Geometry: final body of the model. Coordinates: model frame, mm. A direction names the side the tool comes from. Coordinates: 2 decimals unless noted, no trailing zeros. Write each loop counter-clockwise with the first axis right and the second up, starting at its lowest first coordinate (ties: lowest second). Pieces come first, ordered by that corner, then holes. Notation, with made-up numbers: M 68,22.25 L 83,22.25 A22 cw 83,51.25 Z; hole C 89,66 d11. An arc over 180 degrees is marked long. Write item = value, one per line. Start each with the question number.
Item 1: First-contact query: pin 1 Ø10 at (x, z) = (4, -7.5) entering from -Y; pin 2 Ø8 at (x, z) = (-5, -3) entering from -Y; pin 3 Ø2 at (x, z) = (14.5, 0.5) entering from -Y; pin 4 Ø1.6 at (x, z) = (17, 6) entering from -Y. Flat tips, straight axial feed; report the tip coordinate or a pass-through.
Item 2: Section C-C on x = -9. Output: boundary loops of the cut face in (y, z) (3 decimals).
Item 3: Reachability of faces 4 (the flat face through (0, 2, 0)), 5 (the flat face through (0, 5, 12.925)), 6 (the flat face through (15.72, 0.99, -0.18)) from +Z, -Z, +X, -X, +Y, -Y: full face, straight path, thin tool, end or side. Return the list, or none.
Item 4: Section A-A on y = -3. Give the number of separate pieces and of enclosed holes in the cut face, plus the area to 3 significant figures.
Item 5: Pull-direction query (X, two-part tool) for faces 1 (the flat face through (-15.704, 1.014, -0.181)), 2 (the flat face through (-17.9, 4, 0)), 3 (the flat face through (0, 5, -12.925)); classes: +X half, -X half, draft (parallel to the pull), parting line (faces both ways), or undercut.
Item 6: Ray query, L1, parallel to Y at x = 2, z = -4; L2, parallel to X at y = 1.75, z = 7.75; L3, parallel to X at y = 0.75, z = -4.25. Return the intervals inside material, ascending. Write a range as [from, to].
Item 7: Section B-B on z = -5.75. Output: boundary loops of the cut face in (x, y), plus the area to 3 significant figures.
from build123d import *

# Parameters (mm, degrees)
SKETCH_1_W                  = 35.8
SKETCH_1_H                  = 25.85
EXTRUDE_1_DEPTH             = 7.74
CUT_EXTRUDE_1_DEPTH         = 33.38116891
CUT_EXTRUDE_1_DEPTH_BACK    = 33.38116891
SKETCH_1_4_R                = 0.25
EXTRUDE_2_DEPTH             = 4
EXTRUDE_2_DIRECTION_2_REACH = 25.396


with BuildPart() as part:
    # Sketch 1 → Extrude 1 (new body)
    with BuildSketch(Plane(origin=(0, 0, 0), x_dir=(1, 0, 0), z_dir=(0, 1, 0))):
        Rectangle(SKETCH_1_W, SKETCH_1_H)
    extrude(amount=EXTRUDE_1_DEPTH)

    # Sketch 2 → Cut-Extrude 1 (cut, two sides: drawn at the far end of the back side and taken through both)
    with BuildSketch(Plane.XY.offset(12.925).offset(-CUT_EXTRUDE_1_DEPTH_BACK)):
        Polygon((-15.027609673, 2), (-16.4, 0), (16.4, 0), (15.027609673, 2), align=None)
    extrude(amount=CUT_EXTRUDE_1_DEPTH + CUT_EXTRUDE_1_DEPTH_BACK, mode=Mode.SUBTRACT)

    # Sketch 1_4 → Extrude 2 (add)
    with BuildSketch(Plane(origin=(0, 0, 0), x_dir=(1, 0, 0), z_dir=(0, 1, 0))):
        with Locations((-10.16, -11)):
            Circle(SKETCH_1_4_R)
        with Locations((-7.62, -11)):
            Circle(SKETCH_1_4_R)
        with Locations((-5.08, -11)):
            Circle(SKETCH_1_4_R)
        with Locations((-2.54, -11)):
            Circle(SKETCH_1_4_R)
        with Locations((0, -11)):
            Circle(SKETCH_1_4_R)
        with Locations((2.54, -11)):
            Circle(SKETCH_1_4_R)
        with Locations((5.08, -11)):
            Circle(SKETCH_1_4_R)
        with Locations((7.62, -11)):
            Circle(SKETCH_1_4_R)
        with Locations((10.16, -11)):
            Circle(SKETCH_1_4_R)
        with Locations(Location((10.16, 11, 0), (0, 0, 90))):
            Circle(SKETCH_1_4_R)
        with Locations(Location((7.62, 11, 0), (0, 0, 90))):
            Circle(SKETCH_1_4_R)
        with Locations(Location((5.08, 11, 0), (0, 0, 90))):
            Circle(SKETCH_1_4_R)
        with Locations(Location((2.54, 11, 0), (0, 0, 90))):
            Circle(SKETCH_1_4_R)
        with Locations(Location((0, 11, 0), (0, 0, 90))):
            Circle(SKETCH_1_4_R)
        with Locations(Location((-2.54, 11, 0), (0, 0, 90))):
            Circle(SKETCH_1_4_R)
        with Locations(Location((-5.08, 11, 0), (0, 0, 90))):
            Circle(SKETCH_1_4_R)
        with Locations(Location((-7.62, 11, 0), (0, 0, 90))):
            Circle(SKETCH_1_4_R)
        with Locations(Location((-10.16, 11, 0), (0, 0, 90))):
            Circle(SKETCH_1_4_R)
    extrude(amount=-EXTRUDE_2_DEPTH)

    # Sketch 1_4 → Extrude 2 direction 2 (add, up to next)
    with BuildSketch(Plane(origin=(0, 0, 0), x_dir=(1, 0, 0), z_dir=(0, 1, 0)), mode=Mode.PRIVATE) as extrude_2_direction_2_sk1:
        with Locations((-10.16, -11)):
            Circle(SKETCH_1_4_R)
    extrude_2_direction_2_tool1 = extrude(extrude_2_direction_2_sk1.sketch, amount=EXTRUDE_2_DIRECTION_2_REACH, mode=Mode.PRIVATE) - part.part
    # Sketch 1_4 → Extrude 2 direction 2 (add, up to next)
    with BuildSketch(Plane(origin=(0, 0, 0), x_dir=(1, 0, 0), z_dir=(0, 1, 0)), mode=Mode.PRIVATE) as extrude_2_direction_2_sk2:
        with Locations((-7.62, -11)):
            Circle(SKETCH_1_4_R)
    extrude_2_direction_2_tool2 = extrude(extrude_2_direction_2_sk2.sketch, amount=EXTRUDE_2_DIRECTION_2_REACH, mode=Mode.PRIVATE) - part.part
    # Sketch 1_4 → Extrude 2 direction 2 (add, up to next)
    with BuildSketch(Plane(origin=(0, 0, 0), x_dir=(1, 0, 0), z_dir=(0, 1, 0)), mode=Mode.PRIVATE) as extrude_2_direction_2_sk3:
        with Locations((-5.08, -11)):
            Circle(SKETCH_1_4_R)
    extrude_2_direction_2_tool3 = extrude(extrude_2_direction_2_sk3.sketch, amount=EXTRUDE_2_DIRECTION_2_REACH, mode=Mode.PRIVATE) - part.part
    # Sketch 1_4 → Extrude 2 direction 2 (add, up to next)
    with BuildSketch(Plane(origin=(0, 0, 0), x_dir=(1, 0, 0), z_dir=(0, 1, 0)), mode=Mode.PRIVATE) as extrude_2_direction_2_sk4:
        with Locations((-2.54, -11)):
            Circle(SKETCH_1_4_R)
    extrude_2_direction_2_tool4 = extrude(extrude_2_direction_2_sk4.sketch, amount=EXTRUDE_2_DIRECTION_2_REACH, mode=Mode.PRIVATE) - part.part
    # Sketch 1_4 → Extrude 2 direction 2 (add, up to next)
    with BuildSketch(Plane(origin=(0, 0, 0), x_dir=(1, 0, 0), z_dir=(0, 1, 0)), mode=Mode.PRIVATE) as extrude_2_direction_2_sk5:
        with Locations((0, -11)):
            Circle(SKETCH_1_4_R)
    extrude_2_direction_2_tool5 = extrude(extrude_2_direction_2_sk5.sketch, amount=EXTRUDE_2_DIRECTION_2_REACH, mode=Mode.PRIVATE) - part.part
    # Sketch 1_4 → Extrude 2 direction 2 (add, up to next)
    with BuildSketch(Plane(origin=(0, 0, 0), x_dir=(1, 0, 0), z_dir=(0, 1, 0)), mode=Mode.PRIVATE) as extrude_2_direction_2_sk6:
        with Locations((2.54, -11)):
            Circle(SKETCH_1_4_R)
    extrude_2_direction_2_tool6 = extrude(extrude_2_direction_2_sk6.sketch, amount=EXTRUDE_2_DIRECTION_2_REACH, mode=Mode.PRIVATE) - part.part
    # Sketch 1_4 → Extrude 2 direction 2 (add, up to next)
    with BuildSketch(Plane(origin=(0, 0, 0), x_dir=(1, 0, 0), z_dir=(0, 1, 0)), mode=Mode.PRIVATE) as extrude_2_direction_2_sk7:
        with Locations((5.08, -11)):
            Circle(SKETCH_1_4_R)
    extrude_2_direction_2_tool7 = extrude(extrude_2_direction_2_sk7.sketch, amount=EXTRUDE_2_DIRECTION_2_REACH, mode=Mode.PRIVATE) - part.part
    # Sketch 1_4 → Extrude 2 direction 2 (add, up to next)
    with BuildSketch(Plane(origin=(0, 0, 0), x_dir=(1, 0, 0), z_dir=(0, 1, 0)), mode=Mode.PRIVATE) as extrude_2_direction_2_sk8:
        with Locations((7.62, -11)):
            Circle(SKETCH_1_4_R)
    extrude_2_direction_2_tool8 = extrude(extrude_2_direction_2_sk8.sketch, amount=EXTRUDE_2_DIRECTION_2_REACH, mode=Mode.PRIVATE) - part.part
    # Sketch 1_4 → Extrude 2 direction 2 (add, up to next)
    with BuildSketch(Plane(origin=(0, 0, 0), x_dir=(1, 0, 0), z_dir=(0, 1, 0)), mode=Mode.PRIVATE) as extrude_2_direction_2_sk9:
        with Locations((10.16, -11)):
            Circle(SKETCH_1_4_R)
    extrude_2_direction_2_tool9 = extrude(extrude_2_direction_2_sk9.sketch, amount=EXTRUDE_2_DIRECTION_2_REACH, mode=Mode.PRIVATE) - part.part
    # Sketch 1_4 → Extrude 2 direction 2 (add, up to next)
    with BuildSketch(Plane(origin=(0, 0, 0), x_dir=(1, 0, 0), z_dir=(0, 1, 0)), mode=Mode.PRIVATE) as extrude_2_direction_2_sk10:
        with Locations(Location((10.16, 11, 0), (0, 0, 90))):
            Circle(SKETCH_1_4_R)
    extrude_2_direction_2_tool10 = extrude(extrude_2_direction_2_sk10.sketch, amount=EXTRUDE_2_DIRECTION_2_REACH, mode=Mode.PRIVATE) - part.part
    # Sketch 1_4 → Extrude 2 direction 2 (add, up to next)
    with BuildSketch(Plane(origin=(0, 0, 0), x_dir=(1, 0, 0), z_dir=(0, 1, 0)), mode=Mode.PRIVATE) as extrude_2_direction_2_sk11:
        with Locations(Location((7.62, 11, 0), (0, 0, 90))):
            Circle(SKETCH_1_4_R)
    extrude_2_direction_2_tool11 = extrude(extrude_2_direction_2_sk11.sketch, amount=EXTRUDE_2_DIRECTION_2_REACH, mode=Mode.PRIVATE) - part.part
    # Sketch 1_4 → Extrude 2 direction 2 (add, up to next)
    with BuildSketch(Plane(origin=(0, 0, 0), x_dir=(1, 0, 0), z_dir=(0, 1, 0)), mode=Mode.PRIVATE) as extrude_2_direction_2_sk12:
        with Locations(Location((5.08, 11, 0), (0, 0, 90))):
            Circle(SKETCH_1_4_R)
    extrude_2_direction_2_tool12 = extrude(extrude_2_direction_2_sk12.sketch, amount=EXTRUDE_2_DIRECTION_2_REACH, mode=Mode.PRIVATE) - part.part
    # Sketch 1_4 → Extrude 2 direction 2 (add, up to next)
    with BuildSketch(Plane(origin=(0, 0, 0), x_dir=(1, 0, 0), z_dir=(0, 1, 0)), mode=Mode.PRIVATE) as extrude_2_direction_2_sk13:
        with Locations(Location((2.54, 11, 0), (0, 0, 90))):
            Circle(SKETCH_1_4_R)
    extrude_2_direction_2_tool13 = extrude(extrude_2_direction_2_sk13.sketch, amount=EXTRUDE_2_DIRECTION_2_REACH, mode=Mode.PRIVATE) - part.part
    # Sketch 1_4 → Extrude 2 direction 2 (add, up to next)
    with BuildSketch(Plane(origin=(0, 0, 0), x_dir=(1, 0, 0), z_dir=(0, 1, 0)), mode=Mode.PRIVATE) as extrude_2_direction_2_sk14:
        with Locations(Location((0, 11, 0), (0, 0, 90))):
            Circle(SKETCH_1_4_R)
    extrude_2_direction_2_tool14 = extrude(extrude_2_direction_2_sk14.sketch, amount=EXTRUDE_2_DIRECTION_2_REACH, mode=Mode.PRIVATE) - part.part
    # Sketch 1_4 → Extrude 2 direction 2 (add, up to next)
    with BuildSketch(Plane(origin=(0, 0, 0), x_dir=(1, 0, 0), z_dir=(0, 1, 0)), mode=Mode.PRIVATE) as extrude_2_direction_2_sk15:
        with Locations(Location((-2.54, 11, 0), (0, 0, 90))):
            Circle(SKETCH_1_4_R)
    extrude_2_direction_2_tool15 = extrude(extrude_2_direction_2_sk15.sketch, amount=EXTRUDE_2_DIRECTION_2_REACH, mode=Mode.PRIVATE) - part.part
    # Sketch 1_4 → Extrude 2 direction 2 (add, up to next)
    with BuildSketch(Plane(origin=(0, 0, 0), x_dir=(1, 0, 0), z_dir=(0, 1, 0)), mode=Mode.PRIVATE) as extrude_2_direction_2_sk16:
        with Locations(Location((-5.08, 11, 0), (0, 0, 90))):
            Circle(SKETCH_1_4_R)
    extrude_2_direction_2_tool16 = extrude(extrude_2_direction_2_sk16.sketch, amount=EXTRUDE_2_DIRECTION_2_REACH, mode=Mode.PRIVATE) - part.part
    # Sketch 1_4 → Extrude 2 direction 2 (add, up to next)
    with BuildSketch(Plane(origin=(0, 0, 0), x_dir=(1, 0, 0), z_dir=(0, 1, 0)), mode=Mode.PRIVATE) as extrude_2_direction_2_sk17:
        with Locations(Location((-7.62, 11, 0), (0, 0, 90))):
            Circle(SKETCH_1_4_R)
    extrude_2_direction_2_tool17 = extrude(extrude_2_direction_2_sk17.sketch, amount=EXTRUDE_2_DIRECTION_2_REACH, mode=Mode.PRIVATE) - part.part
    # Sketch 1_4 → Extrude 2 direction 2 (add, up to next)
    with BuildSketch(Plane(origin=(0, 0, 0), x_dir=(1, 0, 0), z_dir=(0, 1, 0)), mode=Mode.PRIVATE) as extrude_2_direction_2_sk18:
        with Locations(Location((-10.16, 11, 0), (0, 0, 90))):
            Circle(SKETCH_1_4_R)
    extrude_2_direction_2_tool18 = extrude(extrude_2_direction_2_sk18.sketch, amount=EXTRUDE_2_DIRECTION_2_REACH, mode=Mode.PRIVATE) - part.part
    add(extrude_2_direction_2_tool1.solids().sort_by_distance((-10.16, 0, 11))[0])
    add(extrude_2_direction_2_tool2.solids().sort_by_distance((-7.62, 0, 11))[0])
    add(extrude_2_direction_2_tool3.solids().sort_by_distance((-5.08, 0, 11))[0])
    add(extrude_2_direction_2_tool4.solids().sort_by_distance((-2.54, 0, 11))[0])
    add(extrude_2_direction_2_tool5.solids().sort_by_distance((0, 0, 11))[0])
    add(extrude_2_direction_2_tool6.solids().sort_by_distance((2.54, 0, 11))[0])
    add(extrude_2_direction_2_tool7.solids().sort_by_distance((5.08, 0, 11))[0])
    add(extrude_2_direction_2_tool8.solids().sort_by_distance((7.62, 0, 11))[0])
    add(extrude_2_direction_2_tool9.solids().sort_by_distance((10.16, 0, 11))[0])
    add(extrude_2_direction_2_tool10.solids().sort_by_distance((10.16, 0, -11))[0])
    add(extrude_2_direction_2_tool11.solids().sort_by_distance((7.62, 0, -11))[0])
    add(extrude_2_direction_2_tool12.solids().sort_by_distance((5.08, 0, -11))[0])
    add(extrude_2_direction_2_tool13.solids().sort_by_distance((2.54, 0, -11))[0])
    add(extrude_2_direction_2_tool14.solids().sort_by_distance((0, 0, -11))[0])
    add(extrude_2_direction_2_tool15.solids().sort_by_distance((-2.54, 0, -11))[0])
    add(extrude_2_direction_2_tool16.solids().sort_by_distance((-5.08, 0, -11))[0])
    add(extrude_2_direction_2_tool17.solids().sort_by_distance((-7.62, 0, -11))[0])
    add(extrude_2_direction_2_tool18.solids().sort_by_distance((-10.16, 0, -11))[0])


solid = part.part
Responses:
q1.pin_1 = -4
q1.pin_2 = 2
q1.pin_3 = 1.31
q1.pin_4 = 0
q2.outline = M 2,-12.925 L 7.74,-12.925 L 7.74,12.925 L 2,12.925 Z
q3.face_4 = -Y
q3.face_5 = +Z, +X, -X, +Y, -Y
q3.face_6 = +Z, -Z, -Y
q4.separate_pieces = 18
q4.enclosed_holes = 0
q4.area = 3.53 mm²
q5.face_1 = undercut
q5.face_2 = -X half
q5.face_3 = draft
q6.L1 = [2, 7.74]
q6.L2 = [-17.9, -15.2], [15.2, 17.9]
q6.L3 = [-17.9, -15.89], [15.89, 17.9]
q7.outline = M -17.9,0 L -16.4,0 L -15.03,2 L 15.03,2 L 16.4,0 L 17.9,0 L 17.9,7.74 L -17.9,7.74 Z
q7.area = 214 mm²
